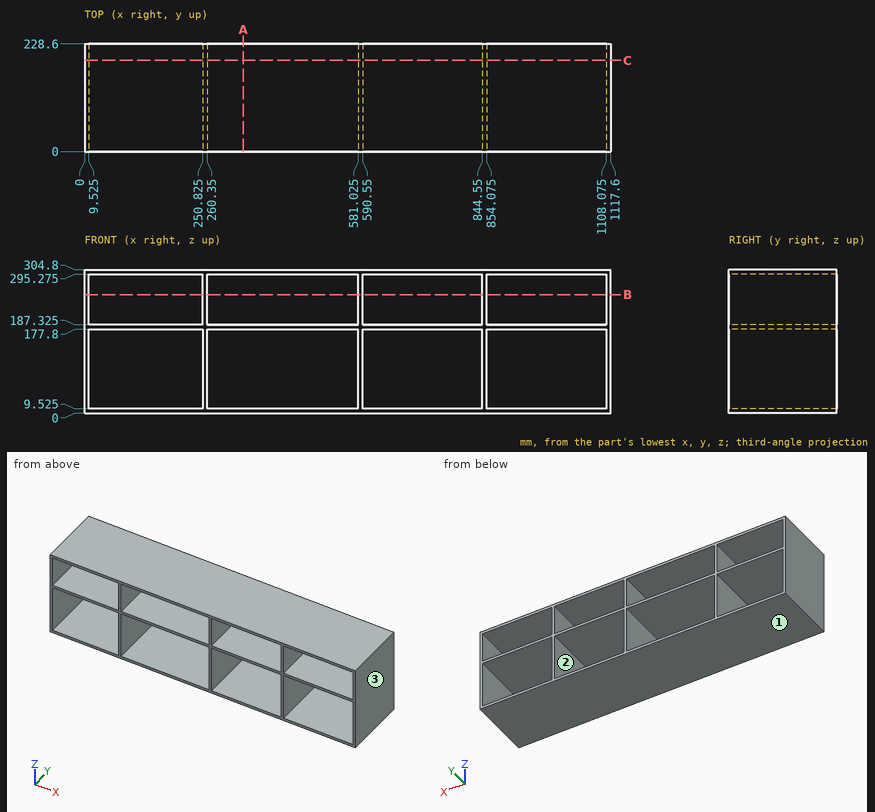
The figure shows three views and two pictorial views of one solid part (mm, origin at its lowest corner). Answer the questions. Coordinates: 2 decimals unless noted, no trailing zeros. Order: outer loops, then holes, each group sorted by start corner. A loop starts at its lowest first (then second) coordinate and runs counter-clockwise, first axis right, second up.
Q1. A cutting plane is placed at B-B, the plane z = 252. Write down the section's boundary in (x, y) (3 decimals), and give its area (3 significant figures).
Q2. A cutting plane is placed at C-C, the plane y = 194. State how many separate pieces and enclosed holes the cut face has, and give its area (3 significant figures).
Q3. Consider line 1 (Z direction, x = 552, y = 219) (3 decimals); line 2 (X direction, y = 100, z = 104) (3 decimals). Determine where each line is inside the solid, lowest interval first.
Q4. A cutting plane is placed at A-A, the plane x = 337.5. Write down the section's boundary in (y, z) (3 decimals).
Q5. For a pull along Z with two mould halves and no side action, classify the marked faces 1, 2 and 3 as pulls with the +Z half, pulls with the -Z half, needs draft (parallel to the pull), parting line crosses it, or undercut.
Answers follow:
1. outline: (0, 0) - (9.525, 0) - (9.525, 228.6) - (0, 228.6) - close; (250.825, 0) - (260.35, 0) - (260.35, 228.6) - (250.825, 228.6) - close; (581.025, 0) - (590.55, 0) - (590.55, 228.6) - (581.025, 228.6) - close; (844.55, 0) - (854.075, 0) - (854.075, 228.6) - (844.55, 228.6) - close; (1108.075, 0) - (1117.6, 0) - (1117.6, 228.6) - (1108.075, 228.6) - close
1. area: 10,900 mm2
2. separate pieces: 1
2. enclosed holes: 8
2. area: 45,100 mm2
3. line 1: z = 0 to 9.525, 177.8 to 187.325, 295.275 to 304.8
3. line 2: x = 0 to 9.525, 250.825 to 260.35, 581.025 to 590.55, 844.55 to 854.075, 1108.075 to 1117.6
4. outline: (0, 0) - (228.6, 0) - (228.6, 9.525) - (0, 9.525) - close; (0, 177.8) - (228.6, 177.8) - (228.6, 187.325) - (0, 187.325) - close; (0, 295.275) - (228.6, 295.275) - (228.6, 304.8) - (0, 304.8) - close
5. face 1: pulls with the -Z half
5. face 2: undercut
5. face 3: needs draft
